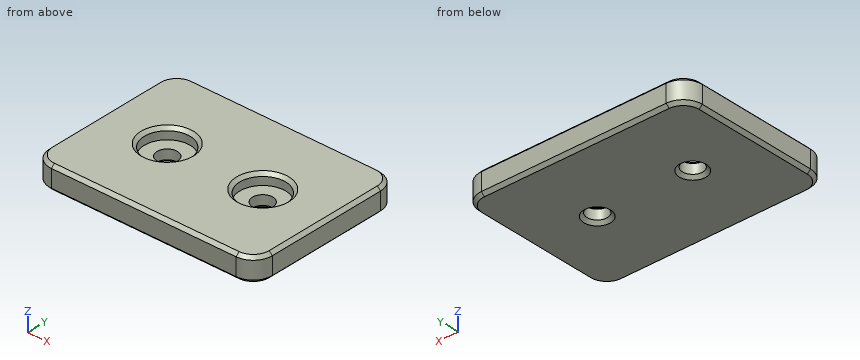
from build123d import *

# Parameters (mm, degrees)
CYLINDER001_R     = 3.6
CYLINDER001_DEPTH = 10
CYLINDER_R        = 1.6
CYLINDER_DEPTH    = 10
BOX_W             = 35
BOX_H             = 25
BOX_DEPTH         = 3.75
FILLET_R          = 3
CHAMFER_SIZE      = 0.5


with BuildPart() as cylinder001:
    # Cylinder001 → Cylinder001 (new body)
    with BuildSketch(Plane(origin=(-7.5, 0, 2), x_dir=(1, 0, 0), z_dir=(0, 0, 1))):
        Circle(CYLINDER001_R)
    extrude(amount=CYLINDER001_DEPTH)


with BuildPart() as fusion:
    # Cylinder → Cylinder (new body)
    with BuildSketch(Plane(origin=(-7.5, 0, -1), x_dir=(1, 0, 0), z_dir=(0, 0, 1))):
        Circle(CYLINDER_R)
    extrude(amount=CYLINDER_DEPTH)

    # Fusion: union Cylinder001
    add(cylinder001.part)


with BuildPart() as part_mirroring:
    # Part__Mirroring: instance of Fusion
    add(fusion.part.mirror(Plane(origin=(0, 0, 0), x_dir=(0, -1, 0), z_dir=(1, 0, 0))))


with BuildPart() as fusion001:
    # Fusion001 base: copy of Fusion
    add(fusion.part)

    # Fusion001: union Part__Mirroring
    add(part_mirroring.part)


with BuildPart() as mountplate:
    # Box → Box (new body)
    with BuildSketch(Plane(origin=(-17.5, -12.5, 0), x_dir=(1, 0, 0), z_dir=(0, 0, 1))):
        with Locations((17.5, 12.5)):
            Rectangle(BOX_W, BOX_H)
    extrude(amount=BOX_DEPTH)

    # Cut001: cut Fusion001
    add(fusion001.part, mode=Mode.SUBTRACT)

    # Fillet
    fillet_edges = [mountplate.edges().sort_by_distance(p)[0] for p in [
        (-17.5, -12.5, 1.875),
        (-17.5, 12.5, 1.875),
        (17.5, -12.5, 1.875),
        (17.5, 12.5, 1.875),
    ]]
    fillet(fillet_edges, radius=FILLET_R)

    # Chamfer
    chamfer_edges = [mountplate.edges().sort_by_distance(p)[0] for p in [
        (-17.5, 0, 3.75),
        (-17.5, 0, 0),
        (-16.62132, -11.62132, 3.75),
        (-16.62132, 11.62132, 3.75),
        (0, -12.5, 3.75),
        (0, 12.5, 3.75),
        (16.62132, -11.62132, 3.75),
        (16.62132, 11.62132, 3.75),
        (17.5, 0, 3.75),
        (-11.1, 0, 3.75),
        (11.1, 0, 3.75),
        (-16.62132, -11.62132, 0),
        (-16.62132, 11.62132, 0),
        (0, -12.5, 0),
        (0, 12.5, 0),
        (16.62132, -11.62132, 0),
        (16.62132, 11.62132, 0),
        (17.5, 0, 0),
        (-9.1, 0, 0),
        (9.1, 0, 0),
    ]]
    chamfer(chamfer_edges, length=CHAMFER_SIZE)


solid = mountplate.part
Source: CAD feature listing. Evaluate the final solid. Frame: model axes, mm. Give positions to 0.01 mm unless a question says otherwise; leave off trailing zeros. Write each loop counter-clockwise with the first axis right and the second up, starting at its lowest first coordinate (ties: lowest second). Pieces come first, ordered by that corner, then holes. Notation, with made-up numbers: (6.25, 3) - (17.25, 3) arc R23 ccw to (17.25, 34) - close; hole circle Ø4 at (20.5, 71). An arc over 180 degrees is marked (long way). Write item = value, one per line. Start each with the question number.
Q1. Cut plane A-A, the plane x = -7.5. Return loops of the section in (y, z).
Q2. Cut plane C-C, the plane z = 2.8. Return loops of the section in (x, y).
Q3. Pin query (flat end, axial travel): pin 1 Ø8.5 at (x, y) = (-7.5, 0) entering from +Z; pin 2 Ø2 at (x, y) = (6, -1) entering from +Z; pin 3 Ø1.9 at (x, y) = (7.5, 0) entering from +Z. Return the tip coordinate at first contact, or that it passes through.
Q4. Material intervals for probe 1 along X at (y, z) = (0, 1.35); probe 2 along X at (y, z) = (-1.25, 2.75); probe 3 along Y at (x, z) = (-7.5, 2.8), sorted ascending.
Q5. Cut plane B-B, the plane y = 0. Give the number of separate pieces and of enclosed holes in the cut face, then the cut area to 4 significant figures.
Computed values:
q1.outline = (-12.5, 0.5) - (-12, 0) - (-2.1, 0) - (-1.6, 0.5) - (-1.6, 2) - (-3.6, 2) - (-3.6, 3.25) - (-4.1, 3.75) - (-12, 3.75) - (-12.5, 3.25) - close; (1.6, 0.5) - (2.1, 0) - (12, 0) - (12.5, 0.5) - (12.5, 3.25) - (12, 3.75) - (4.1, 3.75) - (3.6, 3.25) - (3.6, 2) - (1.6, 2) - close
q2.outline = (-17.5, -9.5) arc R3 ccw to (-14.5, -12.5) - (14.5, -12.5) arc R3 ccw to (17.5, -9.5) - (17.5, 9.5) arc R3 ccw to (14.5, 12.5) - (-14.5, 12.5) arc R3 ccw to (-17.5, 9.5) - close; hole circle Ø7.2 at (-7.5, 0); hole circle Ø7.2 at (7.5, 0)
q3.pin_1 = 3.75
q3.pin_2 = 2
q3.pin_3 = through
q4.probe_1 = -17.5 to -9.1, -5.9 to 5.9, 9.1 to 17.5
q4.probe_2 = -17.5 to -10.88, -4.12 to 4.12, 10.88 to 17.5
q4.probe_3 = -12.5 to -3.6, 3.6 to 12.5
q5.separate_pieces = 3
q5.enclosed_holes = 0
q5.area = 91.75 mm²
